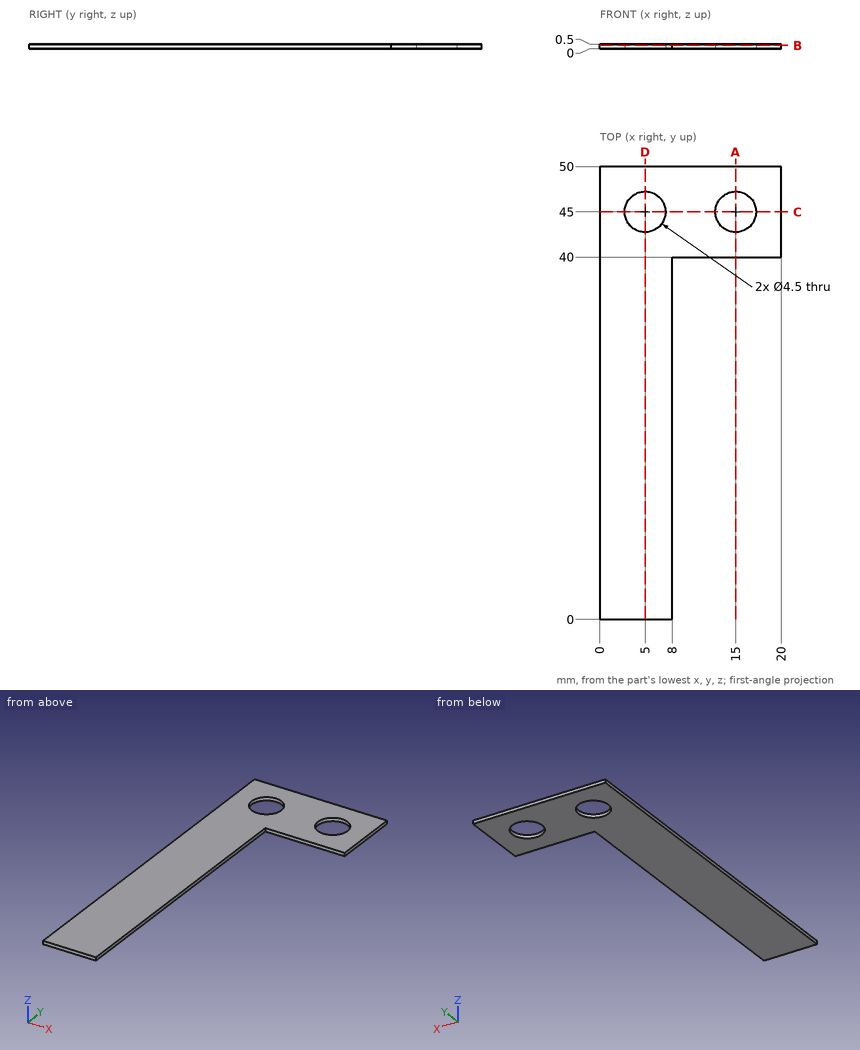
Could you check a few things on this drawing? It's one solid part, dimensions in mm from its lowest x, y, z. Round coordinates to 2 decimals unless told otherwise and drop trailing zeros. Write each loop counter-clockwise with the first axis right and the second up, starting at its lowest first coordinate (ties: lowest second). Pieces come first, ordered by that corner, then holes. Notation, with made-up numbers: M 45.25,25.5 L 84.25,25.5 A31 cw 84.25,51.5 Z; hole C 15.5,38 d7. An arc over 180 degrees is marked long. Answer as CSV lines item,"result". Start each with the question number.
1. I need wall thicknesses on probe 1 along Y at (x, z) = (15, 0.3); probe 2 along Y at (x, z) = (5, 0.35); probe 3 along X at (y, z) = (46, 0.25). Which ranges of each line are inside material? Lowest first, please.
2. Suppose I cut it at C-C on y = 45. Write out the boundary of the cut face in (x, z).
3. Suppose I cut it at B-B on z = 0.35. Write out the boundary of the cut face in (x, y), then the cut area to 3 significant figures.
4. Suppose I cut it at A-A on x = 15. Write out the boundary of the cut face in (y, z), then the cut area to 3 significant figures.
5. Suppose I cut it at D-D on x = 5. Write out the boundary of the cut face in (y, z).
Check result:
1,probe 1,"y = 40 to 42.75, 47.25 to 50"
1,probe 2,"y = 0 to 42.75, 47.25 to 50"
1,probe 3,"x = 0 to 2.98, 7.02 to 12.98, 17.02 to 20"
2,outline,"M 0,0 L 2.75,0 L 2.75,0.5 L 0,0.5 Z; M 7.25,0 L 12.75,0 L 12.75,0.5 L 7.25,0.5 Z; M 17.25,0 L 20,0 L 20,0.5 L 17.25,0.5 Z"
3,outline,"M 0,0 L 8,0 L 8,40 L 20,40 L 20,50 L 0,50 Z; hole C 5,45 d4.5; hole C 15,45 d4.5"
3,area,"488 mm2"
4,outline,"M 40,0 L 42.75,0 L 42.75,0.5 L 40,0.5 Z; M 47.25,0 L 50,0 L 50,0.5 L 47.25,0.5 Z"
4,area,"2.75 mm2"
5,outline,"M 0,0 L 42.75,0 L 42.75,0.5 L 0,0.5 Z; M 47.25,0 L 50,0 L 50,0.5 L 47.25,0.5 Z"
